from build123d import *

# Parameters (mm, degrees)
SKETCH_W        = 60
SKETCH_H        = 60
PAD_DEPTH       = 11.15
SKETCH001_R     = 2.1
SKETCH001_R_2   = 3.2
POCKET_DEPTH    = 12
SKETCH002_R     = 4.2
POCKET001_DEPTH = 3.6


with BuildPart() as part:
    # Sketch → Pad (new body)
    with BuildSketch(Plane.XY):
        with Locations((30, 30)):
            Rectangle(SKETCH_W, SKETCH_H)
    extrude(amount=PAD_DEPTH)

    # Sketch001 (on Face6 of Pad) → Pocket (cut)
    with BuildSketch(Plane.XY.offset(11.15)):
        with Locations((15, 35)):
            Circle(SKETCH001_R)
        with Locations((45, 35)):
            Circle(SKETCH001_R)
        with Locations((15, 25)):
            Circle(SKETCH001_R)
        with Locations((45, 25)):
            Circle(SKETCH001_R)
        with Locations((10, 50)):
            Circle(SKETCH001_R_2)
        with Locations((50, 50)):
            Circle(SKETCH001_R_2)
        with Locations((10, 10)):
            Circle(SKETCH001_R_2)
        with Locations((50, 10)):
            Circle(SKETCH001_R_2)
    extrude(amount=-POCKET_DEPTH, mode=Mode.SUBTRACT)

    # Sketch002 (on Face5 of Pocket) → Pocket001 (cut)
    with BuildSketch(Plane.XY.offset(11.15)):
        with Locations((15, 35)):
            Circle(SKETCH002_R)
        with Locations((45, 35)):
            Circle(SKETCH002_R)
        with Locations((45, 25)):
            Circle(SKETCH002_R)
        with Locations((15, 25)):
            Circle(SKETCH002_R)
    extrude(amount=-POCKET001_DEPTH, mode=Mode.SUBTRACT)


solid = part.part
Geometry check sheet. Reference: the model listing, model coordinates, mm. A direction names the side the tool comes from. Give positions to 0.01 mm unless a question says otherwise; leave off trailing zeros. Order: outer loops, then holes, each group sorted by start corner. A loop starts at its lowest first (then second) coordinate and runs counter-clockwise, first axis right, second up.
1) Material ranges on probe 1 along Y at (x, z) = (15, 2.25); probe 2 along Y at (x, z) = (50, 6.5); probe 3 along X at (y, z) = (35.5, 7), recorded low to high.
Results are:
probe 1: y = 0 to 22.9, 27.1 to 32.9, 37.1 to 60
probe 2: y = 0 to 6.8, 13.2 to 46.8, 53.2 to 60
probe 3: x = 0 to 12.96, 17.04 to 42.96, 47.04 to 60
2) Cross-section at B-B (z = 9). Give the number of separate pieces and of enclosed holes in the cut face, then the cut area to 3 significant figures.
Results are:
separate pieces: 1
enclosed holes: 8
area: 3,250 mm2
3) Tool access check on faces 1 (the cylindrical face through (16.13, 26.77, 3.83)), 2 (the cylindrical face through (10.804, 25.185, 9.375)). Record the directions out of +Z, -Z, +X, -X, +Y, -Y that give a thin tool (end or side, any length) a straight path to the whole face; none if there is none.
Results are:
face 1: +Z, -Z
face 2: +Z
4) Draft check along X on faces 3 (the flat face through (0, 30, 5)), 4 (the cylindrical face through (7.461, 48.053, 5.653)), 5 (the flat face through (60, 30, 5)). Enter one of: released by +X, released by -X, zero draft, split by the parting line, or undercut.
Results are:
face 3: released by -X
face 4: undercut
face 5: released by +X
5) Cross-section at C-C (y = 35). Record the boundary of the cut face in (x, z), then the cut area to 3 significant figures.
Results are:
outline: (0, 0) - (12.9, 0) - (12.9, 7.55) - (10.8, 7.55) - (10.8, 11.15) - (0, 11.15) - close; (17.1, 0) - (42.9, 0) - (42.9, 7.55) - (40.8, 7.55) - (40.8, 11.15) - (19.2, 11.15) - (19.2, 7.55) - (17.1, 7.55) - close; (47.1, 0) - (60, 0) - (60, 11.15) - (49.2, 11.15) - (49.2, 7.55) - (47.1, 7.55) - close
area: 545 mm2
6) Gauge pin test, flat ends, axial feed: pin 1 (4 mm diameter, centred on x = 15, y = 25, fed in from -Z) (3 decimals); pin 2 (4 mm diameter, centred on x = 46.5, y = 36, fed in from +Z). Record the tip position at first contact, or that the pin passes through.
Results are:
pin 1: passes through
pin 2: stops at z = 7.55
7) Cross-section at A-A (x = 10). Record the boundary of the cut face in (y, z), then the cut area to 3 significant figures.
Results are:
outline: (0, 0) - (6.8, 0) - (6.8, 11.15) - (0, 11.15) - close; (13.2, 0) - (46.8, 0) - (46.8, 11.15) - (13.2, 11.15) - close; (53.2, 0) - (60, 0) - (60, 11.15) - (53.2, 11.15) - close
area: 526 mm2
8) Cross-section at D-D (x = 45). Record the boundary of the cut face in (y, z).
Results are:
outline: (0, 0) - (22.9, 0) - (22.9, 7.55) - (20.8, 7.55) - (20.8, 11.15) - (0, 11.15) - close; (27.1, 0) - (32.9, 0) - (32.9, 7.55) - (30.8, 7.55) - (30.8, 11.15) - (29.2, 11.15) - (29.2, 7.55) - (27.1, 7.55) - close; (37.1, 0) - (60, 0) - (60, 11.15) - (39.2, 11.15) - (39.2, 7.55) - (37.1, 7.55) - close
